```python
from build123d import *
from OCP.BRepFilletAPI import BRepFilletAPI_MakeChamfer

# Parameters (mm, degrees)
SKETCH1_R           = 7.25
BOSS_EXTRUDE1_DEPTH = 10
CHAMFER2_SIZE       = 1
CHAMFER2_SIZE2      = 1.732050808


with BuildPart() as part:
    # Sketch1 → Boss-Extrude1 (new, symmetric)
    with BuildSketch(Plane(origin=(0, 0, 0), x_dir=(1, 0, 0), z_dir=(0, 1, 0))):
        Polygon((-12.124355653, 0), (-6.062177826, -10.5), (6.062177826, -10.5), (12.124355653, 0), (6.062177826, 10.5), (-6.062177826, 10.5), align=None)
        with Locations(Location((0, 0, 0), (0, 0, 270))):
            Circle(SKETCH1_R, mode=Mode.SUBTRACT)
    extrude(amount=BOSS_EXTRUDE1_DEPTH, both=True)

    # Chamfer1: read off the stored shape, not the designer's step
    # Chamfer1 outline → Chamfer1 (revolve, cut)
    with BuildSketch(Plane.XY):
        Polygon((7.25, 10), (7.25, 8.5), (8.75, 10), align=None)
    revolve(axis=Axis((0, 0, 0), (0, 1, 0)), mode=Mode.SUBTRACT)

    # Chamfer2: one chamfer whose edges measure the first distance from different faces: ONE call of the kernel's chamfer builder (chamfer() names one face for all edges)
    chamfer2_edges_1 = [part.edges().sort_by_distance(p)[0] for p in [
        (0, 10, 10.5),
    ]]
    chamfer2_side_1 = [part.faces().sort_by_distance(p)[0] for p in [
        (0, 0, 10.5),
    ]]
    chamfer2_edges_2 = [part.edges().sort_by_distance(p)[0] for p in [
        (9.09326674, 10, 5.25),
    ]]
    chamfer2_side_2 = [part.faces().sort_by_distance(p)[0] for p in [
        (9.09326674, 0, 5.25),
    ]]
    chamfer2_edges_3 = [part.edges().sort_by_distance(p)[0] for p in [
        (9.09326674, 10, -5.25),
    ]]
    chamfer2_side_3 = [part.faces().sort_by_distance(p)[0] for p in [
        (9.09326674, 0, -5.25),
    ]]
    chamfer2_edges_4 = [part.edges().sort_by_distance(p)[0] for p in [
        (0, 10, -10.5),
    ]]
    chamfer2_side_4 = [part.faces().sort_by_distance(p)[0] for p in [
        (0, 0, -10.5),
    ]]
    chamfer2_edges_5 = [part.edges().sort_by_distance(p)[0] for p in [
        (-9.09326674, 10, -5.25),
    ]]
    chamfer2_side_5 = [part.faces().sort_by_distance(p)[0] for p in [
        (-9.09326674, 0, -5.25),
    ]]
    chamfer2_edges_6 = [part.edges().sort_by_distance(p)[0] for p in [
        (0, -10, -10.5),
        (9.09326674, -10, -5.25),
        (9.09326674, -10, 5.25),
        (0, -10, 10.5),
        (-9.09326674, -10, 5.25),
        (-9.09326674, -10, -5.25),
    ]]
    chamfer2_side_6 = [part.faces().sort_by_distance(p)[0] for p in [
        (-8.815462852, -10, 5.089609851),
    ]]
    chamfer2_edges_7 = [part.edges().sort_by_distance(p)[0] for p in [
        (-9.09326674, 10, 5.25),
    ]]
    chamfer2_side_7 = [part.faces().sort_by_distance(p)[0] for p in [
        (-9.09326674, 0, 5.25),
    ]]
    chamfer2 = BRepFilletAPI_MakeChamfer(part.part.solid().wrapped)
    for e in chamfer2_edges_1:
        chamfer2.Add(CHAMFER2_SIZE, CHAMFER2_SIZE2, e.wrapped, chamfer2_side_1[0].wrapped)  # the first distance lies on this face
    for e in chamfer2_edges_2:
        chamfer2.Add(CHAMFER2_SIZE, CHAMFER2_SIZE2, e.wrapped, chamfer2_side_2[0].wrapped)  # the first distance lies on this face
    for e in chamfer2_edges_3:
        chamfer2.Add(CHAMFER2_SIZE, CHAMFER2_SIZE2, e.wrapped, chamfer2_side_3[0].wrapped)  # the first distance lies on this face
    for e in chamfer2_edges_4:
        chamfer2.Add(CHAMFER2_SIZE, CHAMFER2_SIZE2, e.wrapped, chamfer2_side_4[0].wrapped)  # the first distance lies on this face
    for e in chamfer2_edges_5:
        chamfer2.Add(CHAMFER2_SIZE, CHAMFER2_SIZE2, e.wrapped, chamfer2_side_5[0].wrapped)  # the first distance lies on this face
    for e in chamfer2_edges_6:
        chamfer2.Add(CHAMFER2_SIZE, CHAMFER2_SIZE2, e.wrapped, chamfer2_side_6[0].wrapped)  # the first distance lies on this face
    for e in chamfer2_edges_7:
        chamfer2.Add(CHAMFER2_SIZE, CHAMFER2_SIZE2, e.wrapped, chamfer2_side_7[0].wrapped)  # the first distance lies on this face
    add(Compound.cast(chamfer2.Shape()), mode=Mode.REPLACE)


solid = part.part
```
The model under review builds one solid part; all positions refer to its coordinate system, in mm. Give positions to 0.01 mm unless a question says otherwise; leave off trailing zeros. Write each loop counter-clockwise with the first axis right and the second up, starting at its lowest first coordinate (ties: lowest second). Pieces come first, ordered by that corner, then holes. Notation, with made-up numbers: (7, 32) - (60, 32) arc R4 cw to (60, 36) - close; hole circle Ø4 at (-4, 86). An arc over 180 degrees is marked (long way). Answer in a Markdown table with one row per item. Add a question column.
1. Wall thickness on line 1 along Z through (x, y) = (0, 2); line 2 along Y through (x, z) = (-0.5, 7.5); line 3 along X through (y, z) = (-0.25, -0.75): over which ranges is each line inside the solid? List them lowest first. Write a range as [from, to].
2. We need section B-B on y = 3.5. Write out the cut boundary in (x, z), then the cut area to 3 significant figures.
3. Draft analysis for pull direction Y (two halves, no side actions). For faces 1 (the flat face through (8.29, 9.51, 4.88)), 2 (the flat face through (8.624, -9.122, 5.077)), 3 (the flat face through (-9.051, 0.487, -5.324)), state which applies: +Y half, -Y half, draft (parallel to the pull), parting line (faces both ways), or undercut.
4. Insertion check: P1, Ø5, axis at x = 9.5, y = -7, coming from the -Z side; P2, Ø1, axis at y = 3, z = -7.5, coming from the -X side. Each pin has a flat end and moves straight along its axis. Give the tip position at first contact, or say it passes through.
5. We need section C-C on x = 9.5. Write out the cut boundary in (y, z).
Ans:
| question | item | result |
|---|---|---|
| 1 | line 1 | z = [-10.5, -7.25], [7.25, 10.5] |
| 1 | line 2 | y = [-10, 8.77] |
| 1 | line 3 | x = [-11.69, -7.21], [7.21, 11.69] |
| 2 | outline | (-12.12, 0) - (-6.06, -10.5) - (6.06, -10.5) - (12.12, 0) - (6.06, 10.5) - (-6.06, 10.5) - close; hole circle Ø14.5 at (0, 0) |
| 2 | area | 217 mm^2 |
| 3 | face 1 | +Y half |
| 3 | face 2 | -Y half |
| 3 | face 3 | draft |
| 4 | P1 | stops at z = -8.88 |
| 4 | P2 | stops at x = -8.08 |
| 5 | outline | (-10, -2.55) - (-8.27, -4.55) - (9, -4.55) - (10, -1.08) - (10, 1.08) - (9, 4.55) - (-8.27, 4.55) - (-10, 2.55) - close |
